Input: part model. Units: mm. Frame: model coordinates. Face numbers are marked on the shaded views. A direction names the side the tool comes from. Give positions to 0.01 mm unless a question says otherwise; leave off trailing zeros. Loops run counter-clockwise (first coordinate to the right, second up) from the corner with the lowest first, then second, coordinate; pieces in that order, holes last. Notation, with made-up numbers: (36.25, 68.25) -> (57.25, 68.25) arc R19 ccw to (57.25, 91.25) -> close; hole circle Ø9 at (55.25, -13.5). An arc over 180 degrees is marked (long way). Use CSV: the item, a comma, the result in double quotes.
```python
from build123d import *

# Parameters (mm, degrees)
EXTRUDE_1_DEPTH          = 2
CUT_EXTRUDE_1_DEPTH      = 27.54241888
CUT_EXTRUDE_1_DEPTH_BACK = 27.54241888
CHAMFER_1_SIZE           = 2


with BuildPart() as part:
    # 草图1 → 凸台-拉伸1 (new, symmetric)
    with BuildSketch(Plane(origin=(0, 0, 0), x_dir=(1, 0, 0), z_dir=(0, 1, 0))):
        Polygon((-18, 13.5), (-18, 8.5), (-22.5, 8.5), (-22.5, -8.5), (-18, -8.5), (-18, -13.5), (18, -13.5), (18, -8.5), (22.5, -8.5), (22.5, 8.5), (18, 8.5), (18, 13.5), align=None)
    extrude(amount=EXTRUDE_1_DEPTH, both=True)

    # 草图2 → 切除-拉伸1 (cut, two sides: drawn at the far end of the back side and taken through both)
    with BuildSketch(Plane(origin=(0, 2, 0), x_dir=(1, 0, 0), z_dir=(0, 1, 0)).offset(-CUT_EXTRUDE_1_DEPTH_BACK)):
        Polygon((0, 3), (8.5, 8.5), (-8.5, 8.5), align=None)
        Polygon((4, 0), (14.045454545, 6.5), (14.045454545, 3.5), (19.045454545, 3.5), (19.045454545, -3.5), (14.045454545, -3.5), (14.045454545, -6.5), align=None)
        Polygon((8.5, -8.5), (-8.5, -8.5), (0, -3), align=None)
        Polygon((-4, 0), (-14.045454545, -6.5), (-14.045454545, -3.5), (-19.045454545, -3.5), (-19.045454545, 3.5), (-14.045454545, 3.5), (-14.045454545, 6.5), align=None)
    extrude(amount=CUT_EXTRUDE_1_DEPTH + CUT_EXTRUDE_1_DEPTH_BACK, mode=Mode.SUBTRACT)

    # 倒角1
    chamfer_1_edges = [part.edges().sort_by_distance(p)[0] for p in [
        (22.5, 0, -8.5),
        (22.5, 0, 8.5),
        (18, 0, 13.5),
        (-18, 0, 13.5),
        (-22.5, 0, 8.5),
        (-22.5, 0, -8.5),
        (-18, 0, -13.5),
        (18, 0, -13.5),
    ]]
    chamfer(chamfer_1_edges, length=CHAMFER_1_SIZE)


solid = part.part
```
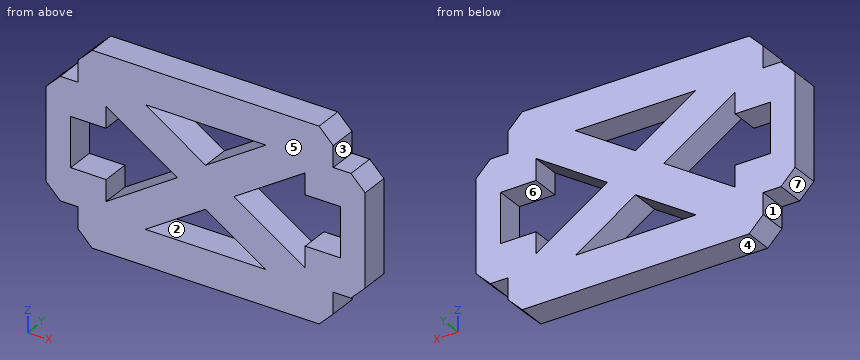
1) Section query B-B (z = 8). Return loops of the section in (x, y), then the cut area to 3 significant figures.
From the geometry:
outline,"(-21, -2) -> (-7.73, -2) -> (-7.73, 2) -> (-21, 2) -> close; (7.73, -2) -> (21, -2) -> (21, 2) -> (7.73, 2) -> close"
area,"106 mm^2"
2) Mould query, pull axis Z, two halves, no side actions, for the marked faces 5, 6 and 7. Classes: pulls with the +Z half, pulls with the -Z half, needs draft (parallel to the pull), parting line crosses it, or undercut.
From the geometry:
face 5,"needs draft"
face 6,"undercut"
face 7,"pulls with the -Z half"
3) Ray query, line 1 (X direction, y = -1.05, z = -5.5); line 2 (X direction, y = -1.4, z = -1.75); line 3 (X direction, y = 0.75, z = 2.5). Return the intervals inside material, ascending.
From the geometry:
line 1,"x = -22.5 to -14.05, -12.5 to -3.86, 3.86 to 12.5, 14.05 to 22.5"
line 2,"x = -22.5 to -19.05, -6.7 to 6.7, 19.05 to 22.5"
line 3,"x = -22.5 to -19.05, -7.86 to 7.86, 19.05 to 22.5"
4) Section query D-D (x = -7). Return loops of the section in (y, z).
From the geometry:
outline,"(-2, -13.5) -> (2, -13.5) -> (2, -8.5) -> (-2, -8.5) -> close; (-2, -7.53) -> (2, -7.53) -> (2, -1.94) -> (-2, -1.94) -> close; (-2, 1.94) -> (2, 1.94) -> (2, 7.53) -> (-2, 7.53) -> close; (-2, 8.5) -> (2, 8.5) -> (2, 13.5) -> (-2, 13.5) -> close"
5) Contact query for flat-ended pins moving along their axis: pin 1 (1.5 mm diameter, centred on y = 0, z = -10, fed in from -X); pin 2 (0.9 mm diameter, centred on y = 0, z = 9.5, fed in from +X); pin 3 (1.2 mm diameter, centred on x = -17.5, y = 0.5, fed in from +Z). Output: stop coordinate, or through.
From the geometry:
pin 1,"stops at x = -18"
pin 2,"stops at x = 18"
pin 3,"stops at z = 12.6"
6) Section query C-C (x = -1.5). Return loops of the section in (y, z), then the cut area to 3 significant figures.
From the geometry:
outline,"(-2, -13.5) -> (2, -13.5) -> (2, -8.5) -> (-2, -8.5) -> close; (-2, -3.97) -> (2, -3.97) -> (2, 3.97) -> (-2, 3.97) -> close; (-2, 8.5) -> (2, 8.5) -> (2, 13.5) -> (-2, 13.5) -> close"
area,"71.8 mm^2"
7) Reachability of the marked faces 1, 2, 3 and 4 from +Z, -Z, +X, -X, +Y, -Y: full face, straight path, thin tool, end or side. Return the list, or none.
From the geometry:
face 1,"-Z, -X, +Y, -Y"
face 2,"+Y, -Y"
face 3,"+Z, +X, +Y, -Y"
face 4,"-Z, +X, -X, +Y, -Y"
8) Section query A-A (x = 16.5). Return loops of the section in (y, z), then the cut area to 3 significant figures.
From the geometry:
outline,"(-2, -13) -> (2, -13) -> (2, -3.5) -> (-2, -3.5) -> close; (-2, 3.5) -> (2, 3.5) -> (2, 13) -> (-2, 13) -> close"
area,"76.0 mm^2"
